Autodesk Inventor part; units mm, degrees
ref_plane "YZ Plane" through (0, 0, 0) normal (1, 0, 0) x (0, 1, 0)
ref_plane "XZ Plane" through (0, 0, 0) normal (0, 1, 0) x (-1, 0, 0)
ref_plane "XY Plane" through (0, 0, 0) normal (0, 0, 1) x (1, 0, 0)
sketch "Sketch1" plane through (0, 0, 0) normal (0, 1, 0) x (-1, 0, 0)
  line L0 (0, 0) -> (0, -25.4)
  line L1 (0, -25.4) -> (3.175, -25.4)
  line L2 (3.175, -25.4) -> (3.175, -3.175)
  line L3 (3.175, -3.175) -> (25.4, -3.175)
  line L4 (25.4, -3.175) -> (25.4, 0)
  line L5 (25.4, 0) -> (0, 0)
  dimension "d0" = 25.4
  dimension "d1" = 3.175
  dimension "d2" = 22.225
  dimension "d3" = 22.225
extrude "Extrusion1" add sketch "Sketch1" along normal blind 50.8
sketch "Sketch2" plane through (-25.4, 0, 0) normal (0, 0, 1) x (1, 0, 0)
  line L0 (22.225, 0) -> (22.225, 50.8)
  line L1 (22.225, 0) -> (0, 0)
  line L2 (22.225, 50.8) -> (0, 50.8)
  circle A0 centre (14.605, 45.72) radius 3.175
  circle A1 centre (14.605, 5.08) radius 3.175
  circle A2 centre (-9.525, 25.4) radius 24.13
  line L3 (25.4, 0) -> (22.225, 0)
  dimension "d9" = 6.35
  dimension "d10" = 6.35
extrude "Extrusion2" cut sketch "Sketch2" against normal blind 63.5
sketch "Sketch3" plane through (0, 0, 0) normal (1, 0, 0) x (0, 0, -1)
  line L0 (25.4, 0) -> (25.4, 50.8)
  line L1 (0, 3.2295) -> (0, 47.5705)
  line L2 (0, 50.8) -> (25.4, 50.8)
  line L3 (25.4, 0) -> (3.175, 0)
  circle A0 centre (12.7, 9.525) radius 3.175
  circle A1 centre (12.7, 41.275) radius 3.175
  point P0 (0, 0)
extrude "Extrusion3" cut sketch "Sketch3" against normal blind 63.5
properties part number "Frame Bracket"
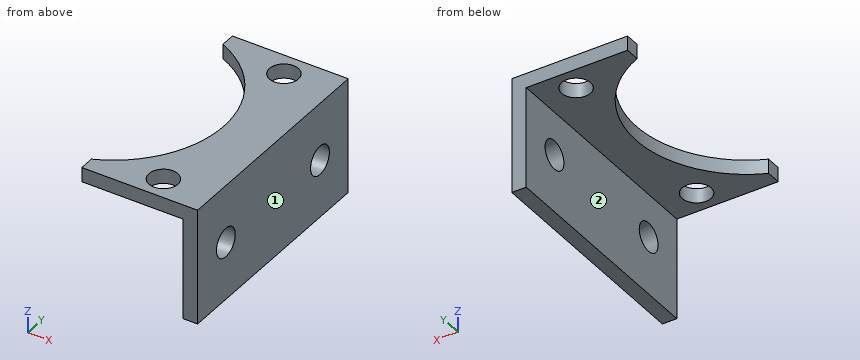
Here's how the part is built. I have some questions about the finished solid (model axes, mm). Face numbers are marked on the shaded views. A direction names the side the tool comes from. Give positions to 0.01 mm unless a question says otherwise; leave off trailing zeros. Write each loop counter-clockwise with the first axis right and the second up, starting at its lowest first coordinate (ties: lowest second). Pieces come first, ordered by that corner, then holes. Notation, with made-up numbers: (68.25, 18.25) -> (125.25, 18.25) arc R8 cw to (125.25, 28.25) -> close; hole circle Ø11 at (7.5, -23.75). An arc over 180 degrees is marked (long way). Write each question's results on one line, items separated by ' | '.
Item 1: If I drill on L1, parallel to Y at x = -2, z = -12.7; L2, parallel to X at y = 23, z = -4.5 (3 decimals), over which ranges is the centre line in solid material (lowest first)?
Output:
L1: y = 0 to 6.35, 12.7 to 38.1, 44.45 to 50.8 | L2: x = -3.175 to 0
Item 2: Suppose I cut it at A-A on z = -11.75. Write out the boundary of the cut face in (x, y) (3 decimals), plus the area to 3 significant figures.
Output:
outline: (-3.175, 0) -> (0, 0) -> (0, 6.495) -> (-3.175, 6.495) -> close; (-3.175, 12.555) -> (0, 12.555) -> (0, 38.245) -> (-3.175, 38.245) -> close; (-3.175, 44.305) -> (0, 44.305) -> (0, 50.8) -> (-3.175, 50.8) -> close | area: 123 mm^2
Item 3: For pin 1 Ø5 at (x, y) = (-10.795, 45.72) entering from -Z; pin 2 Ø6 at (x, y) = (-4.5, 24) entering from +Z; pin 3 Ø10 at (y, z) = (41.275, -12.7) entering from -X (3 decimals); pin 4 Ø8 at (x, y) = (-9.5, 35) entering from -Z (3 decimals), each with a flat end and sliding along its axis, tell me the tip position at first contact or that it passes through.
Output:
pin 1: passes through | pin 2: stops at z = 0 | pin 3: stops at x = -3.175 | pin 4: stops at z = -3.175
Item 4: Suppose I cut it at D-D on z = -14.5. Write out the boundary of the cut face in (x, y) (3 decimals).
Output:
outline: (-3.175, 0) -> (0, 0) -> (0, 6.91) -> (-3.175, 6.91) -> close; (-3.175, 12.14) -> (0, 12.14) -> (0, 38.66) -> (-3.175, 38.66) -> close; (-3.175, 43.89) -> (0, 43.89) -> (0, 50.8) -> (-3.175, 50.8) -> close
Item 5: Suppose I cut it at C-C on y = 45.72. Write out the boundary of the cut face in (x, z) (3 decimals), plus the area to 3 significant figures.
Output:
outline: (-21.911, -3.175) -> (-13.97, -3.175) -> (-13.97, 0) -> (-21.911, 0) -> close; (-7.62, -3.175) -> (-3.175, -3.175) -> (-3.175, -25.4) -> (0, -25.4) -> (0, 0) -> (-7.62, 0) -> close | area: 120 mm^2
Item 6: On a 3-axis mill with a long thin cutter (end or side, diameter ignored), from which of +Z, -Z, +X, -X, +Y, -Y can I reach the whole of each face in a straight line? I mean the marked faces 1 and 2. Say none if no direction works.
Output:
face 1: +Z, -Z, +X, +Y, -Y | face 2: -Z, -X, +Y, -Y
Item 7: Suppose I cut it at B-B on x = -17.25. Write out the boundary of the cut face in (y, z) (3 decimals).
Output:
outline: (0, -3.175) -> (8.973, -3.175) -> (8.973, 0) -> (0, 0) -> close; (41.827, -3.175) -> (50.8, -3.175) -> (50.8, 0) -> (41.827, 0) -> close
